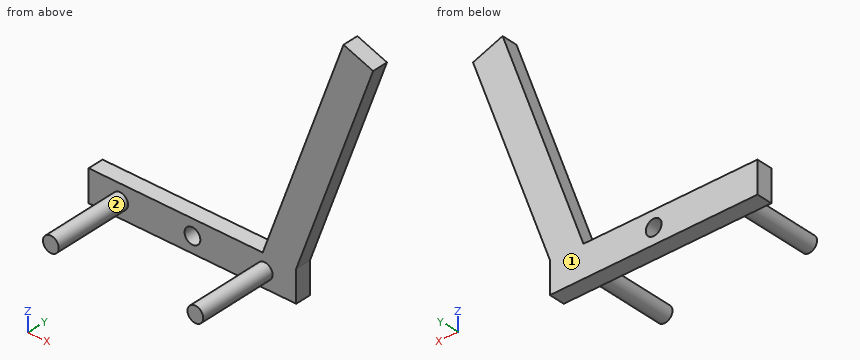
from build123d import *

# Parameters (mm, degrees)
F0_W     = 131.7172
F0_H     = 20
F0_R     = 5
F1_DEPTH = 10
F2_R     = 5
F3_DEPTH = 50
F5_DEPTH = 10


with BuildPart() as f1:
    # F0 (on Front) → F1 (new body)
    with BuildSketch(Plane.XZ):
        Rectangle(F0_W, F0_H)
        Circle(F0_R, mode=Mode.SUBTRACT)
    extrude(amount=F1_DEPTH)

    # F2 (on face) → F3 (join)
    with BuildSketch(Plane.XZ.offset(10)):
        with Locations((-45.8586, 0)):
            Circle(F2_R)
        with Locations((45.8586, 0)):
            Circle(F2_R)
    extrude(amount=F3_DEPTH)

    # F4 (on Front) → F5 (join)
    with BuildSketch(Plane.XZ):
        Polygon((95.878066, 150.953893), (44.575044, 10), (63.368897, 3.159597), (114.671918, 144.11349), align=None)
    extrude(amount=F5_DEPTH)


solid = f1.part
The listing builds one solid part. Answer for the finished solid, in the listing's coordinates (mm). Face numbers are marked on the shaded views. Coordinates: 2 decimals unless noted, no trailing zeros. Loops run counter-clockwise (first coordinate to the right, second up) from the corner with the lowest first, then second, coordinate; pieces in that order, holes last. Notation, with made-up numbers: (9, 51) -> (60, 51) arc R19 cw to (60, 63) -> close; hole circle Ø10 at (44, 53). An arc over 180 degrees is marked (long way). Answer in a Markdown table with one row per item. Add a question column.
1. Flat-ended cylindrical pins translate along their axes: P1, Ø1.5, axis at x = -47.5, y = -47.5, coming from the +Z side; P2, Ø12, axis at x = 53.5, y = -48, coming from the -Z side; P3, Ø3, axis at x = -35, y = -4.5, coming from the +Z side. Find the tip coordinate at first contact, or state that the pin passes through.
2. The part is cut by section A-A, the plane z = 0. Write down the section's boundary in (x, y).
3. The part is cut by section B-B, the plane x = 0. Write down the section's boundary in (y, z).
4. The part is cut by section C-C, the plane y = -6. Write down the section's boundary in (x, z), then the cut area to 3 significant figures.
5. The part is cut by section D-D, the plane y = -41.5. Write down the section's boundary in (x, z), then the cut area to 3 significant figures.
6. Consider line 1 (Z direction, x = 0, y = -6.75); line 2 (Z direction, x = 28.5, y = -6); line 3 (Y direction, x = 95.5, z = 125). Determine where each line is inside the solid, lowest interval first. Write a range as [from, to].
7. Determine the mould class of the marked faces 1 and 2 for opening direction X: +X half, -X half, draft (parallel to the pull), parting line (faces both ways), or undercut.
Answer below:
| question | item | result |
|---|---|---|
| 1 | P1 | z = 4.92 |
| 1 | P2 | z = -4.72 |
| 1 | P3 | z = 10 |
| 2 | outline | (-65.86, -10) -> (-50.86, -10) -> (-50.86, -60) -> (-40.86, -60) -> (-40.86, -10) -> (-5, -10) -> (-5, 0) -> (-65.86, 0) -> close; (5, -10) -> (40.86, -10) -> (40.86, -60) -> (50.86, -60) -> (50.86, -10) -> (65.86, -10) -> (65.86, 0) -> (5, 0) -> close |
| 3 | outline | (-10, -10) -> (0, -10) -> (0, -5) -> (-10, -5) -> close; (-10, 5) -> (0, 5) -> (0, 10) -> (-10, 10) -> close |
| 4 | outline | (-65.86, -10) -> (65.86, -10) -> (65.86, 10) -> (114.67, 144.11) -> (95.88, 150.95) -> (44.58, 10) -> (-65.86, 10) -> close; hole circle Ø10 at (0, 0) |
| 4 | area | 5,480 mm2 |
| 5 | outline | circle Ø10 at (-45.86, 0); circle Ø10 at (45.86, 0) |
| 5 | area | 157 mm2 |
| 6 | line 1 | [-10, -5], [5, 10] |
| 6 | line 2 | [-10, 10] |
| 6 | line 3 | [-10, 0] |
| 7 | face 1 | draft |
| 7 | face 2 | undercut |
